from build123d import *

# Parameters (mm, degrees)
F0_W     = 127
F0_H     = 304.8
F0_R     = 2.286
F0_R_2   = 10.50925
F1_DEPTH = 5.08


with BuildPart() as f1:
    # F0 (on Front) → F1 (new body)
    with BuildSketch(Plane.XZ):
        with Locations((63.5, -152.4)):
            Rectangle(F0_W, F0_H)
        with BuildLine():
            Line((95.25, -266.7), (31.75, -266.7))
            Line((31.75, -266.7), (31.75, -247.65))
            ThreePointArc((31.75, -247.65), (37.329616, -234.179616), (50.8, -228.6))
            Line((50.8, -228.6), (76.2, -228.6))
            ThreePointArc((76.2, -228.6), (89.670384, -234.179616), (95.25, -247.65))
            Line((95.25, -247.65), (95.25, -266.7))
        make_face(mode=Mode.SUBTRACT)
        with Locations((38.989, -38.1)):
            Circle(F0_R, mode=Mode.SUBTRACT)
        with Locations((63.5, -38.1)):
            Circle(F0_R_2, mode=Mode.SUBTRACT)
        with Locations((88.011, -38.1)):
            Circle(F0_R, mode=Mode.SUBTRACT)
    extrude(amount=F1_DEPTH)


solid = f1.part
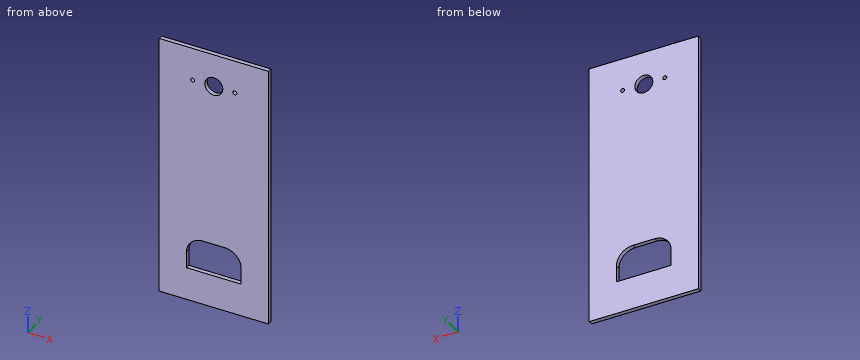
Could you check a few things on this model? Use its own coordinates, in mm. Give positions to 0.01 mm unless a question says otherwise; leave off trailing zeros. Order: outer loops, then holes, each group sorted by start corner. A loop starts at its lowest first (then second) coordinate and runs counter-clockwise, first axis right, second up.
Item 1: If we section it at B-B, the plane z = -30.5: Write out the boundary of the cut face in (x, y).
Item 2: I'm going to push a flat-ended pin straight in: pin 1 (2 mm diameter, centred on y = -3, z = -266.5, fed in from -X). Where does the tip first touch, or does it pass through?
Item 3: If we section it at D-D, the plane x = 47.5: Write out the boundary of the cut face in (y, z), plus the area to 3 significant figures.
Item 4: If we section it at A-A, the plane x = 63.5: Write out the boundary of the cut face in (y, z), plus the area to 3 significant figures.
Item 5: If we section it at C-C, the plane y = -1.2: Count the separate pieces of the cut face and the enclosed holes in it, plus the area to 3 significant figures.
Item 6: I need wall thicknesses on line 1 (Z direction, x = 63.5, y = -1); line 2 (Z direction, x = 59, y = -2.55); line 3 (Z direction, x = 52, y = -4.8). Which ranges of each line are inside material? Lowest first, please.
Values:
1. outline: (0, -5.08) - (56.24, -5.08) - (56.24, 0) - (0, 0) - close; (70.76, -5.08) - (127, -5.08) - (127, 0) - (70.76, 0) - close
2. pin 1: stops at x = 0
3. outline: (-5.08, -304.8) - (0, -304.8) - (0, -266.7) - (-5.08, -266.7) - close; (-5.08, -228.89) - (0, -228.89) - (0, 0) - (-5.08, 0) - close
3. area: 1,360 mm2
4. outline: (-5.08, -304.8) - (0, -304.8) - (0, -266.7) - (-5.08, -266.7) - close; (-5.08, -228.6) - (0, -228.6) - (0, -48.61) - (-5.08, -48.61) - close; (-5.08, -27.59) - (0, -27.59) - (0, 0) - (-5.08, 0) - close
4. area: 1,250 mm2
5. separate pieces: 1
5. enclosed holes: 4
5. area: 36,100 mm2
6. line 1: z = -304.8 to -266.7, -228.6 to -48.61, -27.59 to 0
6. line 2: z = -304.8 to -266.7, -228.6 to -47.6, -28.6 to 0
6. line 3: z = -304.8 to -266.7, -228.6 to 0
